Read the model definition and answer for the solid it produces. Units are mm, in the model's axes. Coordinates: 2 decimals unless noted, no trailing zeros. Order: outer loops, then holes, each group sorted by start corner. A loop starts at its lowest first (then second) coordinate and runs counter-clockwise, first axis right, second up.
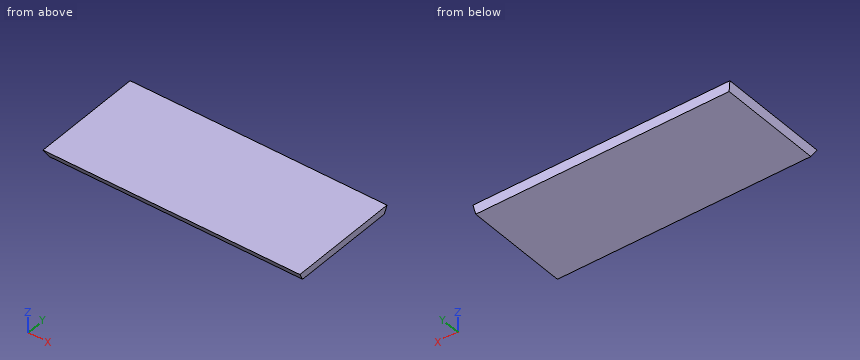
from build123d import *

# Parameters (mm, degrees)
SKETCH1_W           = 107.5
SKETCH1_H           = 23.5
BOSS_EXTRUDE1_DEPTH = 3
CUT_EXTRUDE1_DEPTH  = 109
CUT_EXTRUDE2_DEPTH  = 23.5
SKETCH4_W           = 107.387981152
SKETCH4_H           = 23.388196601
CUT_EXTRUDE3_DEPTH  = 0.1


with BuildPart() as part:
    # Sketch1 → Boss-Extrude1 (new body)
    with BuildSketch(Plane.XY):
        with Locations((53.75, 11.75)):
            Rectangle(SKETCH1_W, SKETCH1_H)
    boss_extrude1 = extrude(amount=BOSS_EXTRUDE1_DEPTH)

    # Sketch2 → Cut-Extrude1 (cut)
    with BuildSketch(Plane(origin=(107.5, 0, 0), x_dir=(0, 0, -1), z_dir=(1, 0, 0))):
        Polygon((-3.423606798, 23.6), (0.1, 21.838196601), (0.1, 23.6), align=None)
    cut_extrude1 = extrude(amount=-CUT_EXTRUDE1_DEPTH, mode=Mode.SUBTRACT)

    # Sketch3 → Cut-Extrude2 (cut)
    with BuildSketch(Plane.XZ):
        Polygon((-0.1, -0.1), (1.661792848, -0.1), (-0.1, 3.424099531), align=None)
    cut_extrude2 = extrude(amount=-CUT_EXTRUDE2_DEPTH, mode=Mode.SUBTRACT)

    # Sketch4 → Cut-Extrude3 (cut)
    with BuildSketch(Plane.XY.offset(3)):
        with Locations((53.806009424, 11.694098301)):
            Rectangle(SKETCH4_W, SKETCH4_H)
    cut_extrude3 = extrude(amount=-CUT_EXTRUDE3_DEPTH, mode=Mode.SUBTRACT)

    # Mirror2: Boss-Extrude1, Cut-Extrude1, Cut-Extrude2, Cut-Extrude3 across plane
    add(boss_extrude1.mirror(Plane(origin=(0, 0, 3), x_dir=(0, 0, 1), z_dir=(0, 1, 0))))
    add(cut_extrude1.mirror(Plane(origin=(0, 0, 3), x_dir=(0, 0, 1), z_dir=(0, 1, 0))), mode=Mode.SUBTRACT)
    add(cut_extrude2.mirror(Plane(origin=(0, 0, 3), x_dir=(0, 0, 1), z_dir=(0, 1, 0))), mode=Mode.SUBTRACT)
    add(cut_extrude3.mirror(Plane(origin=(0, 0, 3), x_dir=(0, 0, 1), z_dir=(0, 1, 0))), mode=Mode.SUBTRACT)


solid = part.part
Q1. The part is cut by section A-A, the plane x = 30. Determine the outline of the cut face in (y, z), then the cut area to 3 significant figures.
Q2. Straight lines are drawn through the part: L1, parallel to X at y = -20, z = 1.85; L2, parallel to X at y = -15, z = 2.55; L3, parallel to Y at x = 91, z = 1. For each, find the intervals that lie inside material, in ascending order.
Q3. This flat-tipped pin is pushed along its axis until it touches: P1, Ø1.5, axis at x = 54.5, z = 1.5, coming from the +Y side. Where does it stop, or does it pass through?
Q4. The part is cut by section B-B, the plane z = 1.05. Determine the outline of the cut face in (x, y).
Computed values:
1. outline: (-23.34, 2.9) - (-21.89, 0) - (21.89, 0) - (23.34, 2.9) - close
1. area: 131 mm2
2. L1: x = 0.69 to 107.5
2. L2: x = 0.34 to 107.5
2. L3: y = -22.39 to 22.39
3. P1: stops at y = 23.01
4. outline: (1.09, -22.41) - (107.5, -22.41) - (107.5, 22.41) - (1.09, 22.41) - close
